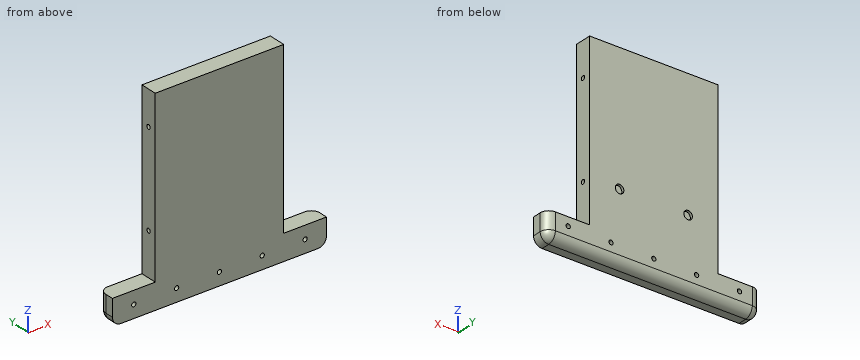
from build123d import *

# Parameters (mm, degrees)
BOSS_EXTRUDE1_DEPTH = 20
SKETCH2_R           = 2.5
CUT_EXTRUDE1_DEPTH  = 240.374184072
SKETCH4_R           = 2.5
CUT_EXTRUDE2_DEPTH  = 5
FILLET1_R           = 10
FILLET2_R           = 10
SKETCH6_R           = 2.5
CUT_EXTRUDE3_DEPTH  = 5
SKETCH8_R           = 5
CUT_EXTRUDE5_DEPTH  = 3


with BuildPart() as part:
    # Sketch1 → Boss-Extrude1 (new body)
    with BuildSketch(Plane(origin=(0, 0, 0), x_dir=(1, 0, 0), z_dir=(0, 1, 0))):
        Polygon((-75, -100), (75, -100), (75, 100), (125, 100), (125, 130), (-125, 130), (-125, 100), (-75, 100), align=None)
    extrude(amount=BOSS_EXTRUDE1_DEPTH)

    # Sketch2 → Cut-Extrude1 (cut, through all)
    with BuildSketch(Plane.ZY.offset(75)):
        with Locations((60, 10)):
            Circle(SKETCH2_R)
        with Locations((-50, 10)):
            Circle(SKETCH2_R)
    extrude(amount=-CUT_EXTRUDE1_DEPTH, mode=Mode.SUBTRACT)

    # Sketch4 → Cut-Extrude2 (cut)
    with BuildSketch(Plane.XZ):
        with Locations(Location((-100, -115, 0), (0, 0, 270))):
            Circle(SKETCH4_R)
        with Locations(Location((-50, -115, 0), (0, 0, 270))):
            Circle(SKETCH4_R)
        with Locations(Location((0, -115, 0), (0, 0, 270))):
            Circle(SKETCH4_R)
        with Locations(Location((50, -115, 0), (0, 0, 90))):
            Circle(SKETCH4_R)
        with Locations(Location((100, -115, 0), (0, 0, 90))):
            Circle(SKETCH4_R)
    extrude(amount=-CUT_EXTRUDE2_DEPTH, mode=Mode.SUBTRACT)

    # Fillet1
    fillet1_edges = [part.edges().sort_by_distance(p)[0] for p in [
        (-125, 10, -130),
        (125, 10, -130),
    ]]
    fillet(fillet1_edges, radius=FILLET1_R)

    # Fillet2
    fillet2_edges = [part.edges().sort_by_distance(p)[0] for p in [
        (125, 20, -110),
        (0, 20, -130),
        (-125, 20, -110),
        (-122.071067812, 20, -127.071067812),
        (122.071067812, 20, -127.071067812),
    ]]
    fillet(fillet2_edges, radius=FILLET2_R)

    # Sketch6 → Cut-Extrude3 (cut)
    with BuildSketch(Plane(origin=(0, 20, 0), x_dir=(1, 0, 0), z_dir=(0, 1, 0))):
        with Locations(Location((0, 110, 0), (0, 0, 270))):
            Circle(SKETCH6_R)
        with Locations(Location((50, 110, 0), (0, 0, 270))):
            Circle(SKETCH6_R)
        with Locations(Location((100, 110, 0), (0, 0, 270))):
            Circle(SKETCH6_R)
        with Locations(Location((-50, 110, 0), (0, 0, 90))):
            Circle(SKETCH6_R)
        with Locations(Location((-100, 110, 0), (0, 0, 90))):
            Circle(SKETCH6_R)
    extrude(amount=-CUT_EXTRUDE3_DEPTH, mode=Mode.SUBTRACT)

    # Sketch8 → Cut-Extrude5 (cut)
    with BuildSketch(Plane(origin=(0, 20, 0), x_dir=(1, 0, 0), z_dir=(0, 1, 0))):
        with Locations(Location((-40, 50, 0), (0, 0, 270))):
            Circle(SKETCH8_R)
        with Locations(Location((40, 50, 0), (0, 0, 90))):
            Circle(SKETCH8_R)
    extrude(amount=-CUT_EXTRUDE5_DEPTH, mode=Mode.SUBTRACT)


solid = part.part
Here's how the part is built. I have some questions about the finished solid (model axes, mm). Coordinates: 2 decimals unless noted, no trailing zeros. Loops run counter-clockwise (first coordinate to the right, second up) from the corner with the lowest first, then second, coordinate; pieces in that order, holes last. Notation, with made-up numbers: (21, 54) -> (48, 54) arc R18 cw to (48, 61) -> close; hole circle Ø4 at (35.5, 28.25). An arc over 180 degrees is marked (long way). Use one line per item in the form item = value. Start each with the question number.
(1) If we section it at A-A (x = -40): Please give me the cut outline in (y, z).
(2) If we section it at B-B (x = -109): Please give me the cut outline in (y, z), then the cut area to 3 significant figures.
(3) Will these pins go through, and if not, where does the flat tip stop? pin 1 (2 mm diameter, centred on y = 9.5, z = -58.5, fed in from +X); pin 2 (2 mm diameter, centred on y = 12.5, z = -104, fed in from +X); pin 3 (1.5 mm diameter, centred on x = -100, z = -111, fed in from +Y); pin 4 (4 mm diameter, centred on x = -1, z = -110, fed in from +Y).
(4) If we section it at C-C (z = -8.5): Please give me the cut outline in (x, y).
(5) Please list where these lines run through material, in increasing order: line 1 along X through (y, z) = (3.1, -115); line 2 along Y through (x, z) = (8, -50); line 3 along X through (y, z) = (16.95, -110).
Verdict:
q1.outline = (0, -130) -> (10, -130) arc R10 ccw to (20, -120) -> (20, -55) -> (17, -55) -> (17, -45) -> (20, -45) -> (20, 100) -> (0, 100) -> close; hole circle Ø5 at (10, -50); hole circle Ø5 at (10, 60)
q2.outline = (0, -130) -> (10, -130) arc R10 ccw to (20, -120) -> (20, -100) -> (0, -100) -> close
q2.area = 579 mm²
q3.pin_1 = 75
q3.pin_2 = 124.89
q3.pin_3 = 15
q3.pin_4 = 20
q4.outline = (-75, 0) -> (75, 0) -> (75, 20) -> (-75, 20) -> close
q5.line_1 = -125 to -102.5, -97.5 to -52.5, -47.5 to -2.5, 2.5 to 47.5, 52.5 to 97.5, 102.5 to 125
q5.line_2 = 0 to 7.5, 12.5 to 20
q5.line_3 = -122.19 to -102.5, -97.5 to -52.5, -47.5 to -2.5, 2.5 to 47.5, 52.5 to 97.5, 102.5 to 122.19
